Source: CAD feature listing. Evaluate the final solid. Frame: model axes, mm. A direction names the side the tool comes from. Round coordinates to 2 decimals unless told otherwise and drop trailing zeros. Order: outer loops, then holes, each group sorted by start corner. A loop starts at its lowest first (then second) coordinate and runs counter-clockwise, first axis right, second up. Notation, with made-up numbers: (44, 15.25) -> (79, 15.25) arc R11 cw to (79, 22.25) -> close; hole circle Ø7 at (76, 24). An arc over 180 degrees is marked (long way). Write item = value, one per line. Start each with the question number.
(1) Reachability of faces 4 (the face through (-20, 0, 3)), 5 (the face through (-17.185, -1.521, -15.695)), 6 (the face through (-2.17, -3.99, -9.76)), 7 (the face through (5, -2, 23)) from +Z, -Z, +X, -X, +Y, -Y: full face, straight path, thin tool, end or side. Return the list, or none.
(2) Cut plane A-A on x = 0. Return the cut outline in (y, z).
(3) Contact query for flat-ended pins moving along their axis: pin 1 Ø1 at (x, y) = (2, 8.5) entering from -Z; pin 2 Ø6 at (y, z) = (1, 7) entering from +X; pin 3 Ø4 at (x, z) = (21.65, -12.5) entering from +Y. Output: stop coordinate, or through.
(4) Ray query, line 1 (X direction, y = -1.75, z = -11.5); line 2 (Y direction, x = 13, z = 4.5); line 3 (X direction, y = 2.25, z = -4). Return the intervals inside material, ascending.
(5) Draft query along X for faces 1 (the face through (-5, -2, 23)), 2 (the face through (22.185, -1.521, -7.035)), 3 (the face through (17.129, -1.521, -15.663)). Return one class per face: released by +X, released by -X, zero draft, split by the parting line, or undercut.
(6) Cut plane C-C on z = -12.5. Return the cut outline in (x, y).
(7) Cut plane B-B on z = 0. Return the cut outline in (x, y), then the cut area to 3 significant figures.
(8) Cut plane D-D on y = 5. Return the cut outline in (x, z), then the cut area to 3 significant figures.
from build123d import *

# Parameters (mm, degrees)
F0_R      = 21
F1_DEPTH  = 3
F2_R      = 3.35
F2_R_2    = 1.8
F3_DEPTH  = 3
F4_R      = 20
F4_R_2    = 17
F5_DEPTH  = 11
F6_R      = 6
F6_R_2    = 5
F7_DEPTH  = 2
F8_R      = 10
F9_DEPTH  = 2
F10_R     = 5
F11_DEPTH = 46.6


with BuildPart() as f1:
    # F0 (on Front) → F1 (new body)
    with BuildSketch(Plane.XZ):
        Circle(F0_R)
    extrude(amount=F1_DEPTH)

    # F2 (on face) → F3 (join)
    with BuildSketch(Plane.XZ.offset(3)):
        with BuildLine():
            Line((5, 20.3960780544), (5, 25))
            ThreePointArc((5, 25), (0, 30), (-5, 25))
            Line((-5, 25), (-5, 20.3960780544))
            ThreePointArc((-5, 20.3960780544), (0, 21), (5, 20.3960780544))
        make_face()
        with Locations((0, 25)):
            Circle(F2_R, mode=Mode.SUBTRACT)
        with BuildLine():
            Line((24.1506350946, -8.1698729811), (20.1635217327, -5.8679120083))
            ThreePointArc((20.1635217327, -5.8679120083), (18.1865334795, -10.5), (15.1635217327, -14.5281660461))
            Line((15.1635217327, -14.5281660461), (19.1506350946, -16.8301270189))
            ThreePointArc((19.1506350946, -16.8301270189), (25.9807621135, -15), (24.1506350946, -8.1698729811))
        make_face()
        with Locations((21.6506350946, -12.5)):
            Circle(F2_R, mode=Mode.SUBTRACT)
        with BuildLine():
            ThreePointArc((-15.1635217327, -14.5281660461), (-18.1865334795, -10.5), (-20.1635217327, -5.8679120083))
            Line((-20.1635217327, -5.8679120083), (-24.1506350946, -8.1698729811))
            ThreePointArc((-24.1506350946, -8.1698729811), (-25.9807621135, -15), (-19.1506350946, -16.8301270189))
            Line((-19.1506350946, -16.8301270189), (-15.1635217327, -14.5281660461))
        make_face()
        with Locations((-21.6506350946, -12.5)):
            Circle(F2_R, mode=Mode.SUBTRACT)
        with Locations((0, 25)):
            Circle(F2_R)
        with Locations((0, 25)):
            Circle(F2_R_2, mode=Mode.SUBTRACT)
        with Locations((-21.6506350946, -12.5)):
            Circle(F2_R)
        with Locations((-21.6506350946, -12.5)):
            Circle(F2_R_2, mode=Mode.SUBTRACT)
        with Locations((21.6506350946, -12.5)):
            Circle(F2_R)
        with Locations((21.6506350946, -12.5)):
            Circle(F2_R_2, mode=Mode.SUBTRACT)
    extrude(amount=-F3_DEPTH)

    # F4 (on face) → F5 (join)
    with BuildSketch(Plane(origin=(0, 0, 0), x_dir=(-1, 0, 0), z_dir=(0, 1, 0))):
        Circle(F4_R)
        Circle(F4_R_2, mode=Mode.SUBTRACT)
    extrude(amount=F5_DEPTH)

    # F6 (on Front) → F7 (join)
    with BuildSketch(Plane.XZ):
        Circle(F6_R)
        Circle(F6_R_2, mode=Mode.SUBTRACT)
        Circle(F6_R_2)
    extrude(amount=-F7_DEPTH)

    # F8 (on face) → F9 (join)
    with BuildSketch(Plane.XZ.offset(3)):
        Circle(F8_R)
    extrude(amount=F9_DEPTH)

    # F10 (on face) → F11 (cut)
    with BuildSketch(Plane(origin=(0, 2, 0), x_dir=(-1, 0, 0), z_dir=(0, 1, 0))):
        Circle(F10_R)
    extrude(amount=-F11_DEPTH, mode=Mode.SUBTRACT)


solid = f1.part
Evaluation:
q1.face_4 = +Y
q1.face_5 = -Z, +Y, -Y
q1.face_6 = -Y
q1.face_7 = +Z, +X, +Y, -Y
q2.outline = (-5, -10) -> (-3, -10) -> (-3, -21) -> (0, -21) -> (0, -20) -> (11, -20) -> (11, -17) -> (0, -17) -> (0, -6) -> (2, -6) -> (2, -5) -> (-5, -5) -> close; (-5, 5) -> (2, 5) -> (2, 6) -> (0, 6) -> (0, 17) -> (11, 17) -> (11, 20) -> (0, 20) -> (0, 23.2) -> (-3, 23.2) -> (-3, 10) -> (-5, 10) -> close; (-3, 26.8) -> (0, 26.8) -> (0, 30) -> (-3, 30) -> close
q3.pin_1 = -19.94
q3.pin_2 = 20.58
q3.pin_3 = 0
q4.line_1 = -26.55 to -23.15, -20.15 to 20.15, 23.15 to 26.55
q4.line_2 = -3 to 0
q4.line_3 = -19.6 to -16.52, 16.52 to 19.6
q5.face_1 = released by -X
q5.face_2 = released by +X
q5.face_3 = undercut
q6.outline = (-26.65, -3) -> (-23.45, -3) -> (-23.45, 0) -> (-26.65, 0) -> close; (-19.85, -3) -> (19.85, -3) -> (19.85, 0) -> (15.61, 0) -> (15.61, 11) -> (11.52, 11) -> (11.52, 0) -> (-11.52, 0) -> (-11.52, 11) -> (-15.61, 11) -> (-15.61, 0) -> (-19.85, 0) -> close; (23.45, -3) -> (26.65, -3) -> (26.65, 0) -> (23.45, 0) -> close
q7.outline = (-21, -3) -> (-10, -3) -> (-10, -5) -> (-5, -5) -> (-5, 2) -> (-6, 2) -> (-6, 0) -> (-17, 0) -> (-17, 11) -> (-20, 11) -> (-20, 0) -> (-21, 0) -> close; (5, -5) -> (10, -5) -> (10, -3) -> (21, -3) -> (21, 0) -> (20, 0) -> (20, 11) -> (17, 11) -> (17, 0) -> (6, 0) -> (6, 2) -> (5, 2) -> close
q7.area = 186 mm^2
q8.outline = circle Ø40 at (0, 0); hole circle Ø34 at (0, 0)
q8.area = 349 mm^2
